Autodesk Inventor part; units mm, degrees
ref_plane "YZ Plane" through (0, 0, 0) normal (1, 0, 0) x (0, 1, 0)
ref_plane "XZ Plane" through (0, 0, 0) normal (0, 1, 0) x (-1, 0, 0)
ref_plane "XY Plane" through (0, 0, 0) normal (0, 0, 1) x (1, 0, 0)
sketch "Sketch1" plane through (0, 0, 0) normal (0, 0, 1) x (1, 0, 0)
  line L0 (0, 0) -> (25.4, 0)
  line L1 (25.4, 0) -> (25.4, 50.8)
  line L2 (25.4, 50.8) -> (0, 50.8)
  line L3 (0, 50.8) -> (0, 0)
  dimension "d0" = 25.4
  dimension "d1" = 50.8
extrude "Extrusion1" add sketch "Sketch1" along normal blind 457.2
shell "Shell1" thickness 2.54 removed faces 2 at (8.4667, 33.8667, 0) at (8.4667, 33.8667, 457.2)
sketch "Sketch2" plane through (0, 50.8, 0) normal (0, 1, 0) x (1, 0, 0)
  line L0 (25.4, 0) -> (0, 0)
  line L1 (0, 0) -> (0, -457.2)
  point P0 (12.7, -12.7)
  point P1 (12.7, -38.1)
  point P2 (12.7, -63.5)
  point P3 (12.7, -88.9)
  point P4 (12.7, -114.3)
  point P5 (12.7, -139.7)
  point P6 (12.7, -165.1)
  point P7 (12.7, -190.5)
  point P8 (12.7, -215.9)
  point P9 (12.7, -241.3)
  point P10 (12.7, -266.7)
  point P11 (12.7, -292.1)
  point P12 (12.7, -317.5)
  point P13 (12.7, -342.9)
  point P14 (12.7, -368.3)
  point P15 (12.7, -393.7)
  point P16 (12.7, -419.1)
  point P17 (12.7, -444.5)
  point P18 (12.7, -469.9)
  point P19 (12.7, -495.3)
  point P20 (12.7, -520.7)
  point P21 (12.7, -546.1)
  point P22 (12.7, -571.5)
  point P23 (12.7, -596.9)
  point P24 (12.7, -622.3)
  point P25 (12.7, -647.7)
  point P26 (12.7, -673.1)
  point P27 (12.7, -698.5)
  point P28 (12.7, -723.9)
  point P29 (12.7, -749.3)
  point P30 (12.7, -774.7)
  dimension "d5" = 12.7
  dimension "d6" = 12.7
  dimension "d9" = 25.4
hole "Hole1" at (12.7, 50.8, 12.7) at (12.7, 50.8, 38.1) at (12.7, 50.8, 63.5) at (12.7, 50.8, 88.9) at (12.7, 50.8, 114.3) at (12.7, 50.8, 139.7) at (12.7, 50.8, 165.1) at (12.7, 50.8, 190.5) at (12.7, 50.8, 215.9) at (12.7, 50.8, 241.3) at (12.7, 50.8, 266.7) at (12.7, 50.8, 292.1) at (12.7, 50.8, 317.5) at (12.7, 50.8, 342.9) at (12.7, 50.8, 368.3) at (12.7, 50.8, 393.7) at (12.7, 50.8, 419.1) at (12.7, 50.8, 444.5) at (12.7, 50.8, 469.9) at (12.7, 50.8, 495.3) at (12.7, 50.8, 520.7) at (12.7, 50.8, 546.1) at (12.7, 50.8, 571.5) at (12.7, 50.8, 596.9) at (12.7, 50.8, 622.3) at (12.7, 50.8, 647.7) at (12.7, 50.8, 673.1) at (12.7, 50.8, 698.5) at (12.7, 50.8, 723.9) at (12.7, 50.8, 749.3) at (12.7, 50.8, 774.7) direction (0, -1, 0) diameter 2.54 depth 50.8 tip angle 118
properties part number "Cross Frame Rail" material "Aluminum 6061"
Source: CAD feature listing. Evaluate the final solid. Frame: model axes, mm. A direction names the side the tool comes from. Coordinates: 2 decimals unless noted, no trailing zeros. Loops run counter-clockwise (first coordinate to the right, second up) from the corner with the lowest first, then second, coordinate; pieces in that order, holes last. Notation, with made-up numbers: M 33,54.5 L 70,54.5 A5 cw 70,62.5 Z; hole C 1,-40 d10. An arc over 180 degrees is marked long. Answer in a Markdown table with one row per item.
Q1. Section A-A on y = 21. Return the cut outline in (x, z).
Answers below:
| item | result |
|---|---|
| outline | M 0,0 L 2.54,0 L 2.54,457.2 L 0,457.2 Z; M 22.86,0 L 25.4,0 L 25.4,457.2 L 22.86,457.2 Z |
Q2. Set-up query: faces 4 (the flat face through (25.4, 25, 225)), 5 (the flat face through (22.86, 25, 225)). Return all of +Z, -Z, +X, -X, +Y, -Y with unobstructed straight access to the full face (end or side cutting, diameter ignored); none if empty.
Answers below:
| item | result |
|---|---|
| face 4 | +Z, -Z, +X, +Y, -Y |
| face 5 | +Z, -Z |
Q3. First-contact query: pin 1 (2 mm diameter, centred on x = 12.7, z = 63.5, fed in from +Y). Flat tip, straight axial feed; report the tip coordinate or a pass-through.
Answers below:
| item | result |
|---|---|
| pin 1 | passes through |
Q4. Section C-C on z = 384.5. Return the cut outline in (x, y).
Answers below:
| item | result |
|---|---|
| outline | M 0,0 L 25.4,0 L 25.4,50.8 L 0,50.8 Z; hole M 2.54,2.54 L 22.86,2.54 L 22.86,48.26 L 2.54,48.26 Z |
Q5. Draft query along X for faces 1 (the flat face through (2, 27, 0)), 2 (the flat face through (13, 48.26, 225)), 3 (the flat face through (0, 26, 225)). Return one class per face: pulls with the +X half, pulls with the -X half, needs draft (parallel to the pull), parting line crosses it, or undercut.
Answers below:
| item | result |
|---|---|
| face 1 | needs draft |
| face 2 | undercut |
| face 3 | pulls with the -X half |
Q6. Section B-B on x = 7.25. Return the cut outline in (y, z), plus the area to 3 significant figures.
Answers below:
| item | result |
|---|---|
| outline | M 0,0 L 2.54,0 L 2.54,457.2 L 0,457.2 Z; M 48.26,0 L 50.8,0 L 50.8,457.2 L 48.26,457.2 Z |
| area | 2,320 mm^2 |
Q7. Ray query, probe 1 along X at (y, z) = (44, 177); probe 2 along Y at (x, z) = (13.25, 162); probe 3 along X at (y, z) = (1.35, 241.3). Return the intervals inside material, ascending. Write a range as from..to.
Answers below:
| item | result |
|---|---|
| probe 1 | x = 0..2.54, 22.86..25.4 |
| probe 2 | y = 0..2.54, 48.26..50.8 |
| probe 3 | x = 0..11.43, 13.97..25.4 |
